Could you check a few things on this model? Use its own coordinates, in mm. A direction names the side the tool comes from. Coordinates: 2 decimals unless noted, no trailing zeros. Write each loop counter-clockwise with the first axis right and the second up, starting at its lowest first coordinate (ties: lowest second). Pieces come first, ordered by that corner, then holes. Notation, with made-up numbers: (19.25, 80.25) - (33.25, 80.25) arc R15 ccw to (33.25, 88.25) - close; hole circle Ø5 at (56.5, 30). An arc over 180 degrees is marked (long way). Answer as a JSON object with one key per item and string values. Group by question number.
1) On a 3-axis mill with a long thin cutter (end or side, diameter ignored), from which of +Z, -Z, +X, -X, +Y, -Y can I reach the whole of each face in a straight line? I mean faces 4 (the flat face through (-76, 60, -10)), 5 (the flat face through (-50, 33, -26.25)), 6 (the cylindrical face through (-30.121, 47.253, -33.029)). Say none if no direction works.
2) If we section it at D-D (z = -28.5): State how many separate pieces and enclosed holes the cut face has, plus the area to 3 significant figures.
3) If we section it at B-B (y = 30): Write out the boundary of the cut face in (x, z), plus the area to 3 significant figures.
4) Please list where these lines run through material, in increasing order: line 1 along X through (y, z) = (50, -23); line 2 along X through (y, z) = (10, -20); line 3 along Y through (x, z) = (-32, -9).
5) If we section it at C-C (x = -50): Write out the boundary of the cut face in (y, z), plus the area to 3 significant figures.
6) We'd pull the mould along X, two halves only. Please class faces 1 (the flat face through (-76, 40, -20)), 2 (the flat face through (-150, 39, -24)), 3 (the flat face through (-70, 13, -6.25)): released by +X, released by -X, zero draft, split by the parting line, or undercut.
7) If we section it at A-A (z = -16): Write out the boundary of the cut face in (x, y), plus the area to 3 significant figures.
8) Will these pins go through, and if not, where does the flat tip stop? pin 1 Ø14.5 at (x, y) = (-30, 30) entering from +Z; pin 2 Ø6.5 at (x, y) = (-70, 70) entering from +Z.
```python
from build123d import *

# Parameters (mm, degrees)
PAD_DEPTH             = 75
SKETCH001_R           = 2.75
POCKET_DEPTH          = 40.001
SKETCH002_R           = 4.5
POCKET001_DEPTH       = 6.25
SKETCH003_R           = 4.5
POCKET002_DEPTH       = 6.25
CLONE_PLACEMENT_ANGLE = 270


with BuildPart() as part:
    # Sketch → Pad (new body, symmetric)
    with BuildSketch(Plane.XZ):
        Polygon((40, 0), (40, -40), (-40, -40), (-40, 0), (-20, 0), (-20, -20), (20, -20), (20, 0), align=None)
    extrude(amount=PAD_DEPTH, both=True)

    # Sketch001 (on Face4 of Pad) → Pocket (cut, through all)
    with BuildSketch(Plane(origin=(0, 0, 0), x_dir=(-1, 0, 0), z_dir=(0, 0, 1))):
        with Locations((-30, -65)):
            Circle(SKETCH001_R)
        with Locations((30, -65)):
            Circle(SKETCH001_R)
        with Locations((-30, -5)):
            Circle(SKETCH001_R)
        with Locations((30, -5)):
            Circle(SKETCH001_R)
        with Locations((-10, -25)):
            Circle(SKETCH001_R)
        with Locations((10, -25)):
            Circle(SKETCH001_R)
        with Locations((-10, -45)):
            Circle(SKETCH001_R)
        with Locations((10, -45)):
            Circle(SKETCH001_R)
    extrude(amount=-POCKET_DEPTH, mode=Mode.SUBTRACT)

    # Sketch002 (on Face16 of Pocket) → Pocket001 (cut)
    with BuildSketch(Plane(origin=(0, 0, 0), x_dir=(-1, 0, 0), z_dir=(0, 0, 1))):
        with Locations((-30, -65)):
            Circle(SKETCH002_R)
        with Locations((-30, -5)):
            Circle(SKETCH002_R)
        with Locations((30, -5)):
            Circle(SKETCH002_R)
        with Locations((30, -65)):
            Circle(SKETCH002_R)
    extrude(amount=-POCKET001_DEPTH, mode=Mode.SUBTRACT)

    # Sketch003 (on Face20 of Pocket001) → Pocket002 (cut)
    with BuildSketch(Plane(origin=(0, 0, -20), x_dir=(-1, 0, 0), z_dir=(0, 0, 1))):
        with Locations((-10, -45)):
            Circle(SKETCH003_R)
        with Locations((-10, -25)):
            Circle(SKETCH003_R)
        with Locations((10, -25)):
            Circle(SKETCH003_R)
        with Locations((10, -45)):
            Circle(SKETCH003_R)
    extrude(amount=-POCKET002_DEPTH, mode=Mode.SUBTRACT)


with BuildPart() as part_1:
    # Clone placement: moved
    add(part.part.moved(Location((-75, 40, 0))).rotate(Axis((-75, 40, 0), (0, 0, 1)), CLONE_PLACEMENT_ANGLE))


solid = part_1.part
```
Here are the results:
{
 "1": {"face 4": "+Z, +X, -X", "face 5": "+Z", "face 6": "+Z, -Z"},
 "2": {"separate pieces": "1", "enclosed holes": "8", "area": "11,800 mm²"},
 "3": {"outline": "(-150, -40) - (-52.75, -40) - (-52.75, -26.25) - (-54.5, -26.25) - (-54.5, -20) - (-150, -20) - close; (-47.25, -40) - (-32.75, -40) - (-32.75, -26.25) - (-34.5, -26.25) - (-34.5, -20) - (-45.5, -20) - (-45.5, -26.25) - (-47.25, -26.25) - close; (-27.25, -40) - (0, -40) - (0, -20) - (-25.5, -20) - (-25.5, -26.25) - (-27.25, -26.25) - close", "area": "2,740 mm²"},
 "4": {"line 1": "x = -150 to -54.5, -45.5 to -34.5, -25.5 to 0", "line 2": "x = -150 to -72.75, -67.25 to -12.75, -7.25 to 0", "line 3": "y = 0 to 20, 60 to 80"},
 "5": {"outline": "(0, -40) - (27.25, -40) - (27.25, -26.25) - (25.5, -26.25) - (25.5, -20) - (20, -20) - (20, 0) - (0, 0) - close; (32.75, -40) - (47.25, -40) - (47.25, -26.25) - (45.5, -26.25) - (45.5, -20) - (34.5, -20) - (34.5, -26.25) - (32.75, -26.25) - close; (52.75, -40) - (80, -40) - (80, 0) - (60, 0) - (60, -20) - (54.5, -20) - (54.5, -26.25) - (52.75, -26.25) - close", "area": "2,140 mm²"},
 "6": {"face 1": "zero draft", "face 2": "released by -X", "face 3": "undercut"},
 "7": {"outline": "(-150, 0) - (0, 0) - (0, 20) - (-150, 20) - close; (-150, 60) - (0, 60) - (0, 80) - (-150, 80) - close; hole circle Ø5.5 at (-70, 10); hole circle Ø5.5 at (-70, 70); hole circle Ø5.5 at (-10, 10); hole circle Ø5.5 at (-10, 70)", "area": "5,900 mm²"},
 "8": {"pin 1": "stops at z = -20", "pin 2": "stops at z = -6.25"}
}
